Source: CAD feature listing. Evaluate the final solid. Frame: model axes, mm. A direction names the side the tool comes from. Give positions to 0.01 mm unless a question says otherwise; leave off trailing zeros. Write each loop counter-clockwise with the first axis right and the second up, starting at its lowest first coordinate (ties: lowest second). Pieces come first, ordered by that corner, then holes. Notation, with made-up numbers: M -32.5,41 L -16.5,41 A24 cw -16.5,66 Z; hole C 17.5,45 d10. An arc over 180 degrees is marked long. Return JSON: item names as keys, results as strings.
```python
from build123d import *

# Parameters (mm, degrees)
SKETCH1_W           = 30
SKETCH1_H           = 30
SKETCH1_W_2         = 27
SKETCH1_H_2         = 27
BOSS_EXTRUDE1_DEPTH = 250
SKETCH2_R           = 2.1
CUT_EXTRUDE1_DEPTH  = 254.574446662


with BuildPart() as part:
    # Sketch1 → Boss-Extrude1 (new body)
    with BuildSketch(Plane.XY):
        with Locations((15, 15)):
            Rectangle(SKETCH1_W, SKETCH1_H)
        with Locations((15, 15)):
            Rectangle(SKETCH1_W_2, SKETCH1_H_2, mode=Mode.SUBTRACT)
    extrude(amount=BOSS_EXTRUDE1_DEPTH)

    # Sketch2 → Cut-Extrude1 (cut, through all)
    with BuildSketch(Plane.ZY):
        with Locations((125, 25)):
            Circle(SKETCH2_R)
        with Locations((125, 5)):
            Circle(SKETCH2_R)
        with Locations((168, 25)):
            Circle(SKETCH2_R)
        with Locations((168, 5)):
            Circle(SKETCH2_R)
        with Locations((82, 5)):
            Circle(SKETCH2_R)
        with Locations((82, 25)):
            Circle(SKETCH2_R)
    extrude(amount=-CUT_EXTRUDE1_DEPTH, mode=Mode.SUBTRACT)


solid = part.part
```
1) Set-up query: faces 1 (the face through (29.24, 5.09, 79.9)), 2 (the face through (15, 1.5, 123)). Return all of +Z, -Z, +X, -X, +Y, -Y with unobstructed straight access to the full face (end or side cutting, diameter ignored); none if empty.
Numbers:
{"face 1": "+X, -X", "face 2": "+Z, -Z"}
2) Cut plane C-C, the plane z = 125. Return the cut outline in (x, y), then the cut area to 3 significant figures.
Numbers:
{"outline": "M 0,0 L 30,0 L 30,2.9 L 28.5,2.9 L 28.5,1.5 L 1.5,1.5 L 1.5,2.9 L 0,2.9 Z; M 0,7.1 L 1.5,7.1 L 1.5,22.9 L 0,22.9 Z; M 0,27.1 L 1.5,27.1 L 1.5,28.5 L 28.5,28.5 L 28.5,27.1 L 30,27.1 L 30,30 L 0,30 Z; M 28.5,7.1 L 30,7.1 L 30,22.9 L 28.5,22.9 Z", "area": "146 mm²"}
3) Cut plane B-B, the plane x = 8.25. Return the cut outline in (y, z).
Numbers:
{"outline": "M 0,0 L 1.5,0 L 1.5,250 L 0,250 Z; M 28.5,0 L 30,0 L 30,250 L 28.5,250 Z"}
4) Line query: line 1 (Y direction, x = 0.45, z = 125); line 2 (Y direction, x = 5, z = 54.5). Output: solid intervals per line, ascending. Write a range as [from, to].
Numbers:
{"line 1": "y = [0, 2.9], [7.1, 22.9], [27.1, 30]", "line 2": "y = [0, 1.5], [28.5, 30]"}
5) Cut plane A-A, the plane y = 25. Give the number of separate pieces and of enclosed holes in the cut face, then the cut area to 3 significant figures.
Numbers:
{"separate pieces": "8", "enclosed holes": "0", "area": "712 mm²"}
6) Draft query along Y for faces 3 (the face through (0, 15, 123)), 4 (the face through (29.24, 25.631, 170.003)), 5 (the face through (15, 30, 123)). Return one class per face: released by +Y, released by -Y, zero draft, split by the parting line, or undercut.
Numbers:
{"face 3": "zero draft", "face 4": "undercut", "face 5": "released by +Y"}
7) Contact query for flat-ended pins moving along their axis: pin 1 Ø3.5 at (y, z) = (5, 82) entering from +X; pin 2 Ø6.5 at (y, z) = (25, 82) entering from +X. Output: stop coordinate, or through.
Numbers:
{"pin 1": "passes through", "pin 2": "stops at x = 30"}
8) Cut plane D-D, the plane z = 219.5. Return the cut outline in (x, y), then the cut area to 3 significant figures.
Numbers:
{"outline": "M 0,0 L 30,0 L 30,30 L 0,30 Z; hole M 1.5,1.5 L 28.5,1.5 L 28.5,28.5 L 1.5,28.5 Z", "area": "171 mm²"}
